Could you check a few things on this model? Use its own coordinates, in mm. Face numbers are marked on the shaded views. A direction names the side the tool comes from. Round coordinates to 2 decimals unless told otherwise and drop trailing zeros. Loops run counter-clockwise (first coordinate to the right, second up) from the corner with the lowest first, then second, coordinate; pieces in that order, holes last. Notation, with made-up numbers: (32.25, -1) -> (72.25, -1) arc R14 cw to (72.25, 11) -> close; hole circle Ø11 at (9, 37.25). An arc over 180 degrees is marked (long way). Put each result on its own line as item: value. Start each with the question number.
1. I'm going to push flat-ended pins straight in: P1, Ø2, axis at x = -2, z = 10.5, coming from the -Y side; P2, Ø3, axis at y = 18, z = 30.5, coming from the +X side; P3, Ø2, axis at y = 19.5, z = 25, coming from the -X side. Where does each tip first touch, or does it pass through?
2. If we mould it in two halves opening along Z, with no side actions, what happens to the marked faces 5, 6, 7 and 8? For each: pulls with the +Z half, pulls with the -Z half, needs draft (parallel to the pull), parting line crosses it, or undercut.
3. Which directions (+Z, -Z, +X, -X, +Y, -Y) give clear straight access to the entire face, cutting with the end or side of a thin tool? Please do the marked faces 1, 2, 3 and 4.
4. Imagine slicing it at B-B, the plane y = 7.35. Please give me the cut outline in (x, z), and give its area (3 significant figures).
5. Imagine slicing it at C-C, the plane x = 6.5. Please give me the cut outline in (y, z), and give its area (3 significant figures).
6. Imagine slicing it at A-A, the plane z = 28.95. Please give me the cut outline in (x, y), and give its area (3 significant figures).
7. I need wall thicknesses on line 1 (Z direction, x = 3.75, y = 18); line 2 (Z direction, x = -1.25, y = 19.75); line 3 (Z direction, x = -0.5, y = 19.5). Which ranges of each line are inside material? Lowest first, please. Write a range as [from, to].
8. Imagine slicing it at D-D, the plane y = 11. Please give me the cut outline in (x, z).
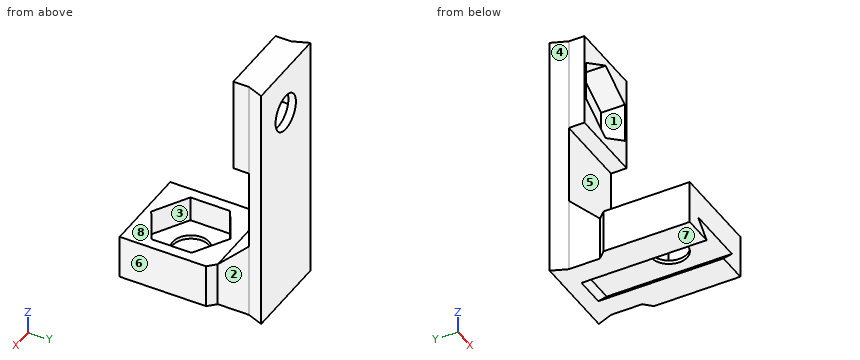
```python
from build123d import *

# Parameters (mm, degrees)
SKETCH1_W               = 12
SKETCH1_H               = 7
BOSS_EXTRUDE1_DEPTH     = 20
CUT_EXTRUDE1_DEPTH      = 20
CUT_EXTRUDE2_REACH      = 24.023
SKETCH3_R               = 2.9
CUT_EXTRUDE3_DEPTH      = 4
SKETCH5_W               = 14
SKETCH5_H               = 40
BOSS_EXTRUDE2_DEPTH     = 2.5
CUT_EXTRUDE4_REACH      = 48.425
SKETCH14_W              = 12
SKETCH14_H              = 15.2
BOSS_EXTRUDE6_DEPTH     = 2.5
CUT_EXTRUDE6_DEPTH      = 2.5
CUT_EXTRUDE6_DEPTH_BACK = 1.3
CUT_EXTRUDE7_REACH      = 44.836
SKETCH9_R               = 2.9
SKETCH10_W              = 1.2
SKETCH10_H              = 7
BOSS_EXTRUDE3_DEPTH     = 15
CHAMFER1_SIZE           = 1.2
SKETCH12_W              = 12
SKETCH12_H              = 5
BOSS_EXTRUDE5_DEPTH     = 10
CHAMFER3_SIZE           = 10


# Some blends are built 0.0001 mm under size
with BuildPart() as part:
    # Sketch1 → Boss-Extrude1 (new body)
    with BuildSketch(Plane(origin=(0, 0, 0), x_dir=(1, 0, 0), z_dir=(0, 1, 0))):
        Rectangle(SKETCH1_W, SKETCH1_H)
    extrude(amount=BOSS_EXTRUDE1_DEPTH)

    # Sketch2 → Cut-Extrude1 (cut)
    with BuildSketch(Plane(origin=(0, 20, 0), x_dir=(1, 0, 0), z_dir=(0, 1, 0))):
        Polygon((0, 3.5), (2.4, 3.5), (4.8, 1.1), (0, 1.1), (-4.8, 1.1), (-2.4, 3.5), align=None)
    extrude(amount=-CUT_EXTRUDE1_DEPTH, mode=Mode.SUBTRACT)

    # Sketch3 → Cut-Extrude2 (cut, up to next)
    with BuildSketch(Plane.XY.offset(3.5), mode=Mode.PRIVATE) as cut_extrude2_sk1:
        with Locations((0, 7.35)):
            Circle(SKETCH3_R)
    cut_extrude2_tool1 = extrude(cut_extrude2_sk1.sketch, amount=-CUT_EXTRUDE2_REACH, mode=Mode.PRIVATE) & part.part
    add(cut_extrude2_tool1.solids().sort_by_distance((0, 7.35, 3.5))[0], mode=Mode.SUBTRACT)

    # Sketch4 → Cut-Extrude3 (cut)
    with BuildSketch(Plane.XY.offset(3.5)):
        Polygon((0, 13.700852961), (-5.5, 10.525426481), (-5.5, 4.174573519), (0, 0.999147039), (5.5, 4.174573519), (5.5, 10.525426481), align=None)
    extrude(amount=-CUT_EXTRUDE3_DEPTH, mode=Mode.SUBTRACT)

    # Sketch5 → Boss-Extrude2 (add)
    with BuildSketch(Plane(origin=(0, 20, 0), x_dir=(1, 0, 0), z_dir=(0, 1, 0))):
        with Locations((0, -16.5)):
            Rectangle(SKETCH5_W, SKETCH5_H)
    extrude(amount=BOSS_EXTRUDE2_DEPTH)

    # Sketch6 → Cut-Extrude4 (cut, up to next)
    with BuildSketch(Plane(origin=(0, 0, -3.5), x_dir=(-1, 0, 0), z_dir=(0, 0, -1)), mode=Mode.PRIVATE) as cut_extrude4_sk1:
        Polygon((-7, 20), (-7, 22.5), (-6, 20), align=None)
    cut_extrude4_tool1 = extrude(cut_extrude4_sk1.sketch, amount=-CUT_EXTRUDE4_REACH, mode=Mode.PRIVATE) & part.part
    # Sketch6 → Cut-Extrude4 (cut, up to next)
    with BuildSketch(Plane(origin=(0, 0, -3.5), x_dir=(-1, 0, 0), z_dir=(0, 0, -1)), mode=Mode.PRIVATE) as cut_extrude4_sk2:
        Polygon((7, 20), (6, 20), (7, 22.5), align=None)
    cut_extrude4_tool2 = extrude(cut_extrude4_sk2.sketch, amount=-CUT_EXTRUDE4_REACH, mode=Mode.PRIVATE) & part.part
    add(cut_extrude4_tool1.solids().sort_by_distance((6.666667, 20.833333, -3.5))[0], mode=Mode.SUBTRACT)
    add(cut_extrude4_tool2.solids().sort_by_distance((-6.666667, 20.833333, -3.5))[0], mode=Mode.SUBTRACT)

    # Sketch14 → Boss-Extrude6 (add)
    with BuildSketch(Plane.XZ.offset(-20)):
        with Locations((0, 28.9)):
            Rectangle(SKETCH14_W, SKETCH14_H)
    extrude(amount=BOSS_EXTRUDE6_DEPTH)

    # Sketch8 → Cut-Extrude6 (cut, two sides: drawn at the far end of the back side and taken through both)
    with BuildSketch(Plane.XZ.offset(-20).offset(-CUT_EXTRUDE6_DEPTH_BACK)):
        Polygon((0, 22.599147039), (5.5, 25.774573519), (5.5, 32.125426481), (0, 35.300852961), (-5.5, 32.125426481), (-5.5, 25.774573519), align=None)
    extrude(amount=CUT_EXTRUDE6_DEPTH + CUT_EXTRUDE6_DEPTH_BACK, mode=Mode.SUBTRACT)

    # Sketch9 → Cut-Extrude7 (cut, up to next)
    with BuildSketch(Plane(origin=(0, 21.3, 0), x_dir=(-1, 0, 0), z_dir=(0, -1, 0)), mode=Mode.PRIVATE) as cut_extrude7_sk1:
        with Locations(Location((0, -28.95, 0), (0, 0, 90))):
            Circle(SKETCH9_R)
    cut_extrude7_tool1 = extrude(cut_extrude7_sk1.sketch, amount=-CUT_EXTRUDE7_REACH, mode=Mode.PRIVATE) & part.part
    add(cut_extrude7_tool1.solids().sort_by_distance((0, 21.3, 28.95))[0], mode=Mode.SUBTRACT)

    # Sketch10 → Boss-Extrude3 (add)
    with BuildSketch(Plane.XZ):
        with Locations((-6.6, 0)):
            Rectangle(SKETCH10_W, SKETCH10_H)
        with Locations((6.6, 0)):
            Rectangle(SKETCH10_W, SKETCH10_H)
    extrude(amount=-BOSS_EXTRUDE3_DEPTH)

    # Chamfer1
    chamfer1_edges = [part.edges().sort_by_distance(p)[0] for p in [
        (7.2, 15, 0),
        (-7.2, 15, 0),
    ]]
    chamfer(chamfer1_edges, length=CHAMFER1_SIZE - 0.0001)  # a hair under: the kernel refuses the full size

    # Sketch12 → Boss-Extrude5 (add)
    with BuildSketch(Plane.XY.offset(3.5)):
        with Locations((0, 17.5)):
            Rectangle(SKETCH12_W, SKETCH12_H)
    extrude(amount=BOSS_EXTRUDE5_DEPTH)

    # Chamfer3
    # the kernel refuses this chamfer: 10 mm, written as the material it takes off along each edge
    with BuildSketch(Plane(origin=(31.71682988, 15, 13.5), x_dir=(0, -0.027495876610586317, -0.9996219169112968), z_dir=(-1, 0, 0))) as chamfer3_piece_1_section:
        Polygon((CHAMFER3_SIZE * 0.999621916911, -CHAMFER3_SIZE * 0.0274958766106), (-CHAMFER3_SIZE * 0.0274958766106, -CHAMFER3_SIZE * 0.999621916911), (0, 0), align=None)
    chamfer3_piece_1 = extrude(amount=63.433659759, mode=Mode.PRIVATE)
    chamfer3_piece_1 = split(chamfer3_piece_1, bisect_by=Plane(origin=(4.860757505, 20, 8.732154153), z_dir=(0, -1, 0)), keep=Keep.TOP, mode=Mode.PRIVATE)
    add(chamfer3_piece_1, mode=Mode.SUBTRACT)


solid = part.part
```
Entries:
1. P1: y = 20
1. P2: x = 6
1. P3: x = -6.2
2. face 5: undercut
2. face 6: needs draft
2. face 7: pulls with the -Z half
2. face 8: pulls with the +Z half
3. face 1: -Y
3. face 2: +Z, -Z, +X
3. face 3: +Z
3. face 4: +Z, -Z, -X
4. outline: (-7.2, -3.5) -> (-2.4, -3.5) -> (-4.8, -1.1) -> (-2.9, -1.1) -> (-2.9, -0.5) -> (-5.5, -0.5) -> (-5.5, 3.5) -> (-7.2, 3.5) -> close; (2.4, -3.5) -> (7.2, -3.5) -> (7.2, 3.5) -> (5.5, 3.5) -> (5.5, -0.5) -> (2.9, -0.5) -> (2.9, -1.1) -> (4.8, -1.1) -> close
4. area: 36.0 mm^2
5. outline: (0, -3.5) -> (14.5, -3.5) -> (14.5, 3.5) -> (0, 3.5) -> close; (21.25, -3.5) -> (22.5, -3.5) -> (22.5, 36.5) -> (21.25, 36.5) -> close
5. area: 152 mm^2
6. outline: (-7, 22.5) -> (-6, 20) -> (-6, 17.5) -> (-5.5, 17.5) -> (-5.5, 21.3) -> (-2.9, 21.3) -> (-2.9, 22.5) -> close; (2.9, 21.3) -> (5.5, 21.3) -> (5.5, 17.5) -> (6, 17.5) -> (6, 20) -> (7, 22.5) -> (2.9, 22.5) -> close
6. area: 13.7 mm^2
7. line 1: [-3.5, -2.15], [-1.1, 6.5], [21.3, 24.76], [33.14, 36.5]
7. line 2: [-1.1, 8.25], [21.3, 23.32], [34.58, 36.5]
7. line 3: [-1.1, 8], [21.3, 22.89], [35.01, 36.5]
8. outline: (-7.2, -3.5) -> (-2.4, -3.5) -> (-4.8, -1.1) -> (4.8, -1.1) -> (2.4, -3.5) -> (7.2, -3.5) -> (7.2, 3.5) -> (4.68, 3.5) -> (4.68, -0.5) -> (-4.68, -0.5) -> (-4.68, 3.5) -> (-7.2, 3.5) -> close
